```python
from build123d import *

# Parameters (mm, degrees)
EXTRUDE_1_DEPTH       = 51.5
SKETCH_2_W            = 49.5
SKETCH_2_H            = 17.5
CUT_EXTRUDE_1_DEPTH   = 10
SKETCH_3_W            = 47.5
SKETCH_3_H            = 1.5
EXTRUDE_2_DEPTH       = 77.5
SKETCH_4_W            = 30
SKETCH_4_H            = 40
EXTRUDE_3_DEPTH       = 14
SKETCH_5_W            = 8
SKETCH_5_H            = 6.2
CUT_EXTRUDE_2_DEPTH   = 24
CHAMFER_1_SIZE        = 2
HOLE_WIZARD_M31_D     = 2.5
HOLE_WIZARD_M31_DEPTH = 8.5
HOLE_WIZARD_M31_TIP   = 0.751075774


with BuildPart() as part:
    # Эскиз1 → Бобышка-Вытянуть1 (new body)
    with BuildSketch(Plane.XY):
        Polygon((1, 1), (77.5, 1), (77.5, 28.5), (78.5, 28.5), (78.5, 0), (0, 0), (0, 28.5), (1, 28.5), align=None)
    extrude(amount=EXTRUDE_1_DEPTH)

    # Эскиз2 → Вырез-Вытянуть1 (cut)
    with BuildSketch(Plane.ZY):
        with Locations((25.75, 9.75)):
            Rectangle(SKETCH_2_W, SKETCH_2_H)
    extrude(amount=-CUT_EXTRUDE_1_DEPTH, mode=Mode.SUBTRACT)

    # Эскиз3 → Бобышка-Вытянуть2 (add)
    with BuildSketch(Plane.ZY.offset(-77.5)):
        with Locations((25.75, 3.25)):
            Rectangle(SKETCH_3_W, SKETCH_3_H)
    extrude(amount=EXTRUDE_2_DEPTH)

    # Эскиз4 → Бобышка-Вытянуть3 (add)
    with BuildSketch(Plane(origin=(0, 4, 0), x_dir=(1, 0, 0), z_dir=(0, 1, 0))):
        with Locations((0, -22)):
            Rectangle(SKETCH_4_W, SKETCH_4_H)
    extrude(amount=EXTRUDE_3_DEPTH)

    # Эскиз5 → Вырез-Вытянуть2 (cut)
    with BuildSketch(Plane(origin=(0, 18, 0), x_dir=(1, 0, 0), z_dir=(0, 1, 0))):
        with Locations((-11, -6.6)):
            Rectangle(SKETCH_5_W, SKETCH_5_H)
        with Locations((-11, -37.4)):
            Rectangle(SKETCH_5_W, SKETCH_5_H)
        with Locations((-11, -14.3)):
            Rectangle(SKETCH_5_W, SKETCH_5_H)
        with Locations((-11, -22)):
            Rectangle(SKETCH_5_W, SKETCH_5_H)
        with Locations((-11, -29.7)):
            Rectangle(SKETCH_5_W, SKETCH_5_H)
    extrude(amount=-CUT_EXTRUDE_2_DEPTH, mode=Mode.SUBTRACT)

    # Фаска1
    chamfer_1_edges = [part.edges().sort_by_distance(p)[0] for p in [
        (-7, 4, 14.3),
        (-7, 18, 14.3),
        (-7, 4, 22),
        (-7, 18, 22),
        (-7, 4, 29.7),
        (-7, 18, 29.7),
        (-7, 4, 37.4),
        (-7, 18, 37.4),
        (-7, 4, 6.6),
        (-7, 18, 6.6),
    ]]
    chamfer(chamfer_1_edges, length=CHAMFER_1_SIZE)

    # Отверстие обработанное метчиком M31
    with Locations(Plane(origin=(0, 0, 0), x_dir=(-1, 0, 0), z_dir=(0, -1, 0))):
        with Locations((-13, -25.4), (-68, -25.4)):
            Hole(HOLE_WIZARD_M31_D / 2, depth=HOLE_WIZARD_M31_DEPTH)
            with Locations((0, 0, -(HOLE_WIZARD_M31_DEPTH + HOLE_WIZARD_M31_TIP / 2))):  # 118° drill point
                Cone(0, HOLE_WIZARD_M31_D / 2, HOLE_WIZARD_M31_TIP, mode=Mode.SUBTRACT)


solid = part.part
```
Check sheet for the modelled part. Datum: model origin and axes. Units: mm. A direction names the side the tool comes from. Give positions to 0.01 mm unless a question says otherwise; leave off trailing zeros. Order: outer loops, then holes, each group sorted by start corner. A loop starts at its lowest first (then second) coordinate and runs counter-clockwise, first axis right, second up. Notation, with made-up numbers: M 21.25,-4.75 L 56.25,-4.75 A21 ccw 56.25,30.25 Z; hole C 15,85 d10. An arc over 180 degrees is marked long. Answer in a Markdown table with one row per item.
1) Cross-section at C-C, the plane x = 26.5. Enter the section's corners in (y, z), plus the area to 3 significant figures.
Filled sheet:
| item | result |
|---|---|
| outline | M 0,0 L 1,0 L 1,51.5 L 0,51.5 Z; M 2.5,2 L 4,2 L 4,49.5 L 2.5,49.5 Z |
| area | 123 mm2 |
2) Cross-section at D-D, the plane y = 15. Count the separate pieces of the cut face and the enclosed holes in it, plus the area to 3 significant figures.
Filled sheet:
| item | result |
|---|---|
| separate pieces | 4 |
| enclosed holes | 0 |
| area | 1,010 mm2 |
3) Release check for a two-part mould opening along X. For faces 1 (the flat face through (1, 22, 24)), 2 (the flat face through (-6, 17, 7)), 3 (the flat face through (-11, 11, 9.7)) record: +X half, -X half, draft (parallel to the pull), parting line (faces both ways), or undercut.
Filled sheet:
| item | result |
|---|---|
| face 1 | undercut |
| face 2 | -X half |
| face 3 | draft |
4) Cross-section at B-B, the plane z = 23. Enter the section's corners in (x, y).
Filled sheet:
| item | result |
|---|---|
| outline | M -7,6 L -5,4 L 0,4 L 0,2.5 L 77.5,2.5 L 77.5,1 L 0,1 L 0,0 L 78.5,0 L 78.5,28.5 L 77.5,28.5 L 77.5,4 L 15,4 L 15,18 L -5,18 L -7,16 Z; M 0,18.5 L 1,18.5 L 1,28.5 L 0,28.5 Z |
5) Thickness scan on L1, parallel to X at y = 3.2, z = 25.4; L2, parallel to X at y = 6.8, z = 25.4; L3, parallel to X at y = 20, z = 5. Record the ranges inside material, lowest first. Write a range as [from, to].
Filled sheet:
| item | result |
|---|---|
| L1 | x = [0, 11.75], [14.25, 66.75], [69.25, 78.5] |
| L2 | x = [-15, 11.75], [14.25, 15], [77.5, 78.5] |
| L3 | x = [0, 1], [77.5, 78.5] |
6) Cross-section at A-A, the plane x = 68. Enter the section's corners in (y, z).
Filled sheet:
| item | result |
|---|---|
| outline | M 0,0 L 1,0 L 1,24.15 L 0,24.15 Z; M 0,26.65 L 1,26.65 L 1,51.5 L 0,51.5 Z; M 2.5,2 L 4,2 L 4,24.15 L 2.5,24.15 Z; M 2.5,26.65 L 4,26.65 L 4,49.5 L 2.5,49.5 Z |
7) Access from +Z, -Z, +X, -X, +Y, -Y to the whole of each face (thin tool, end or side, straight path). Record for faces 4 (the flat face through (-7, 11, 30)), 5 (the flat face through (40, 0, 25)), 6 (the flat face through (-6, 5, 37)).
Filled sheet:
| item | result |
|---|---|
| face 4 | -X, +Y, -Y |
| face 5 | +Z, -Z, +X, -X, -Y |
| face 6 | -X, -Y |
8) Gauge pin test, flat ends, axial feed: P1, Ø8, axis at x = 11, y = 10.5, coming from the -Z side; P2, Ø2, axis at x = 68, z = 25.4, coming from the -Y side; P3, Ø1.9, axis at y = 10.5, z = 23, coming from the -X side; P4, Ø11, axis at x = -10.5, y = 8, coming from the +Z side. Record the tip position at first contact, or that the pin passes through.
Filled sheet:
| item | result |
|---|---|
| P1 | stops at z = 2 |
| P2 | passes through |
| P3 | stops at x = -7 |
| P4 | stops at z = 42 |
